from build123d import *

# Parameters (mm, degrees)
F0_W     = 40
F0_H     = 10
F1_DEPTH = 3
F2_R     = 4
F3_DEPTH = 1
F4_R     = 2
F5_DEPTH = 25
F6_R     = 4.99999


# Not quite as in the source:
# - a fillet or chamfer is up to 0.001 mm smaller than in the source, because OpenCascade refuses the exact size


with BuildPart() as f1:
    # F0 (on Top) → F1 (new body)
    with BuildSketch(Plane.XY):
        Rectangle(F0_W, F0_H)
    extrude(amount=F1_DEPTH)

    # F2 (on face) → F3 (cut)
    with BuildSketch(Plane.XY.offset(3)):
        Circle(F2_R)
    extrude(amount=-F3_DEPTH, mode=Mode.SUBTRACT)

    # F4 (on Top) → F5 (cut)
    with BuildSketch(Plane.XY):
        with Locations((-7.5, 0)):
            Circle(F4_R)
        with Locations((7.5, 0)):
            Circle(F4_R)
        with Locations((-15, 0)):
            Circle(F4_R)
        with Locations((15, 0)):
            Circle(F4_R)
    extrude(amount=F5_DEPTH, mode=Mode.SUBTRACT)

    # F6 (radius 5 in the source; OpenCascade refuses exactly that, so slightly less here)
    f6_edges = [f1.edges().sort_by_distance(p)[0] for p in [
        (-20, -5, 1.5),
        (-20, 5, 1.5),
        (20, -5, 1.5),
        (20, 5, 1.5),
    ]]
    fillet(f6_edges, radius=F6_R)


solid = f1.part
The listing builds one solid part. Answer for the finished solid, in the listing's coordinates (mm). A direction names the side the tool comes from. Round coordinates to 2 decimals unless told otherwise and drop trailing zeros. Write each loop counter-clockwise with the first axis right and the second up, starting at its lowest first coordinate (ties: lowest second). Pieces come first, ordered by that corner, then holes. Notation, with made-up numbers: (81.5, -5.75) - (92.5, -5.75) arc R18 ccw to (92.5, 0.25) - close; hole circle Ø10 at (1, 6). An arc over 180 degrees is marked (long way). Use a Markdown table: item, result. Add a question column.
1. A tool of negligible diameter and unlimited length cuts with its end or side. For faces 5 (the face through (-19, 3, 2)), 6 (the face through (0, 0, 2)), from which of +Z, -Z, +X, -X, +Y, -Y can it reach the whole face along a straight path? Write none if from no direction.
2. The part is cut by section B-B (x = 7.5). Write down the section's boundary in (y, z).
3. The part is cut by section C-C (y = 1). Write down the section's boundary in (x, z), and give its area (3 significant figures).
4. For a pull along Y with two mould halves and no side action, classify faces 1 (the face through (-9.498, 0.088, 1.479)), 2 (the face through (0, -5, 1)), 3 (the face through (13.4, -1.2, 1.5)), 4 (the face through (0, 5, 1)) as +Y half, -Y half, draft (parallel to the pull), parting line (faces both ways), or undercut.
5. The part is cut by section D-D (x = 0). Write down the section's boundary in (y, z).
6. A flat-ended cylindrical pin translates along its axis: P1, Ø1, axis at y = -3, z = 1, coming from the -X side. Find the tip coordinate at first contact, or state that the pin passes through.
7. Consider line 1 (Y direction, x = 15, z = 2.3); line 2 (X direction, y = 0, z = 1.4); line 3 (Y direction, x = 0, z = 2.5). Determine where each line is inside the solid, lowest interval first.
8. The part is cut by section A-A (z = 1). Give the number of separate pieces and of enclosed holes in the cut face, and give its area (3 significant figures).
Reported:
| question | item | result |
|---|---|---|
| 1 | face 5 | +Z, -Z, -X, +Y |
| 1 | face 6 | +Z |
| 2 | outline | (-5, 0) - (-2, 0) - (-2, 3) - (-5, 3) - close; (2, 0) - (5, 0) - (5, 3) - (2, 3) - close |
| 3 | outline | (-19.9, 0) - (-16.73, 0) - (-16.73, 3) - (-19.9, 3) - close; (-13.27, 0) - (-9.23, 0) - (-9.23, 3) - (-13.27, 3) - close; (-5.77, 0) - (5.77, 0) - (5.77, 3) - (3.87, 3) - (3.87, 2) - (-3.87, 2) - (-3.87, 3) - (-5.77, 3) - close; (9.23, 0) - (13.27, 0) - (13.27, 3) - (9.23, 3) - close; (16.73, 0) - (19.9, 0) - (19.9, 3) - (16.73, 3) - close |
| 3 | area | 70.1 mm^2 |
| 4 | face 1 | undercut |
| 4 | face 2 | -Y half |
| 4 | face 3 | undercut |
| 4 | face 4 | +Y half |
| 5 | outline | (-5, 0) - (5, 0) - (5, 3) - (4, 3) - (4, 2) - (-4, 2) - (-4, 3) - (-5, 3) - close |
| 6 | P1 | x = -19.33 |
| 7 | line 1 | -5 to -2, 2 to 5 |
| 7 | line 2 | -20 to -17, -13 to -9.5, -5.5 to 5.5, 9.5 to 13, 17 to 20 |
| 7 | line 3 | -5 to -4, 4 to 5 |
| 8 | separate pieces | 1 |
| 8 | enclosed holes | 4 |
| 8 | area | 328 mm^2 |
